The listing builds one solid part. Answer for the finished solid, in the listing's coordinates (mm). A direction names the side the tool comes from. Coordinates: 2 decimals unless noted, no trailing zeros. Order: outer loops, then holes, each group sorted by start corner. A loop starts at its lowest first (then second) coordinate and runs counter-clockwise, first axis right, second up. Notation, with made-up numbers: (29.25, 83.5) -> (83.25, 83.5) arc R12 ccw to (83.25, 103.5) -> close; hole circle Ø1 at (-32.5, 24.25). An arc over 180 degrees is marked (long way). Answer in a Markdown table with one row per item. Add a question column.
```python
from build123d import *

# Parameters (mm, degrees)
SKETCH1_R           = 65
SKETCH1_R_2         = 40
BOSS_EXTRUDE1_DEPTH = 13
SKETCH2_R           = 4.1
CUT_EXTRUDE1_DEPTH  = 93.838569571
SKETCH8_R           = 12
SKETCH8_R_2         = 4.1
BOSS_EXTRUDE4_DEPTH = 13
SKETCH3_W           = 15.2
SKETCH3_H           = 40
SKETCH3_W_2         = 40
SKETCH3_H_2         = 15.2
CUT_EXTRUDE2_DEPTH  = 10.2
BOSS_EXTRUDE2_DEPTH = 13
FILLET1_R           = 30
BOSS_EXTRUDE3_START = -13
BOSS_EXTRUDE3_DEPTH = 13
CUT_EXTRUDE3_DEPTH  = 93.838569571
FILLET2_R           = 30
SKETCH7_OUTSIDE_W   = 168.862
SKETCH7_OUTSIDE_H   = 168.862
CUT_EXTRUDE4_DEPTH  = 93.838569571
FILLET3_R           = 40


with BuildPart() as part:
    # Sketch1 → Boss-Extrude1 (new body)
    with BuildSketch(Plane(origin=(0, 0, 0), x_dir=(1, 0, 0), z_dir=(0, 1, 0))):
        with Locations(Location((0, 0, 0), (0, 0, 90))):
            Circle(SKETCH1_R)
        with Locations(Location((0, 0, 0), (0, 0, 90))):
            Circle(SKETCH1_R_2, mode=Mode.SUBTRACT)
    extrude(amount=BOSS_EXTRUDE1_DEPTH)

    # Sketch2 → Cut-Extrude1 (cut, through all)
    with BuildSketch(Plane(origin=(0, 13, 0), x_dir=(1, 0, 0), z_dir=(0, 1, 0))):
        with Locations(Location((0, 47, 0), (0, 0, 270))):
            Circle(SKETCH2_R)
        with Locations(Location((47, 0, 0), (0, 0, 270))):
            Circle(SKETCH2_R)
        with Locations(Location((0, -47, 0), (0, 0, 270))):
            Circle(SKETCH2_R)
        with Locations(Location((-47, 0, 0), (0, 0, 270))):
            Circle(SKETCH2_R)
    extrude(amount=-CUT_EXTRUDE1_DEPTH, mode=Mode.SUBTRACT)

    # Sketch8 → Boss-Extrude4 (add)
    # profile 1 of 4: a face of its own
    with BuildSketch(Plane(origin=(0, 13, 0), x_dir=(1, 0, 0), z_dir=(0, 1, 0))):
        with Locations((47, 0)):
            Circle(SKETCH8_R)
        with Locations(Location((47, 0, 0), (0, 0, 270))):
            Circle(SKETCH8_R_2, mode=Mode.SUBTRACT)
    # profile 2 of 4: a face of its own
    with BuildSketch(Plane(origin=(0, 13, 0), x_dir=(1, 0, 0), z_dir=(0, 1, 0))):
        with Locations((0, -47)):
            Circle(SKETCH8_R)
        with Locations(Location((0, -47, 0), (0, 0, 270))):
            Circle(SKETCH8_R_2, mode=Mode.SUBTRACT)
    # profile 3 of 4: a face of its own
    with BuildSketch(Plane(origin=(0, 13, 0), x_dir=(1, 0, 0), z_dir=(0, 1, 0))):
        with Locations((-47, 0)):
            Circle(SKETCH8_R)
        with Locations(Location((-47, 0, 0), (0, 0, 270))):
            Circle(SKETCH8_R_2, mode=Mode.SUBTRACT)
    # profile 4 of 4: a face of its own
    with BuildSketch(Plane(origin=(0, 13, 0), x_dir=(1, 0, 0), z_dir=(0, 1, 0))):
        with Locations((0, 47)):
            Circle(SKETCH8_R)
        with Locations(Location((0, 47, 0), (0, 0, 270))):
            Circle(SKETCH8_R_2, mode=Mode.SUBTRACT)
    extrude(amount=-BOSS_EXTRUDE4_DEPTH)

    # Sketch3 → Cut-Extrude2 (cut)
    with BuildSketch(Plane.XZ):
        with Locations((0, 59.6)):
            Rectangle(SKETCH3_W, SKETCH3_H)
        with Locations((59.6, 0)):
            Rectangle(SKETCH3_W_2, SKETCH3_H_2)
        with Locations((0, -59.6)):
            Rectangle(SKETCH3_W, SKETCH3_H)
        with Locations((-59.6, 0)):
            Rectangle(SKETCH3_W_2, SKETCH3_H_2)
    extrude(amount=-CUT_EXTRUDE2_DEPTH, mode=Mode.SUBTRACT)

    # Sketch4 → Boss-Extrude2 (add)
    with BuildSketch(Plane(origin=(0, 13, 0), x_dir=(1, 0, 0), z_dir=(0, 1, 0))):
        Polygon((-33.587572106, -58.336309448), (-58.336309448, -33.587572106), (-56.639196695, -31.890459353), (-31.890459353, -56.639196695), align=None)
    extrude(amount=-BOSS_EXTRUDE2_DEPTH)

    # Fillet1
    # the kernel refuses this fillet: 30 mm, written as the material it adds along each edge
    with BuildSketch(Plane(origin=(-56.639196695, 13, 31.890459353), x_dir=(-0.43072276652908487, 0, -0.9024842926021104), z_dir=(0, -1, 0))) as fillet1_piece_1:
        with BuildLine():
            CenterArc((10.793469922, -29.931661034), FILLET1_R, 93.868064257, 18.866970785)
            Line((-0.800632502, -2.262602703), (-1.032514551, -1.709221536))
            ThreePointArc((-1.032514551, -1.709221536), (-0.965948102, -0.931149887), (-0.565631851, 0.200151465))
            Line((-0.565631851, 0.200151465), (0.040475512, 0.598633221))
            ThreePointArc((0.040475512, 0.598633221), (4.384847156, 0.451932241), (8.729218799, 0.598633221))
            Line((8.729218799, 0.598633221), (8.769694312, 0))
        make_face()
    extrude(amount=13)
    with BuildSketch(Plane(origin=(-31.890459353, 13, 56.639196695), x_dir=(0.9024842926021067, 0, 0.4307227665290924), z_dir=(0, -1, 0))) as fillet1_piece_2:
        with BuildLine():
            CenterArc((10.793469922, 29.931661034), FILLET1_R, 247.264964958, 18.866970785)
            Line((-0.800632502, 2.262602703), (-1.032514551, 1.709221536))
            ThreePointArc((-1.032514551, 1.709221536), (-0.965948102, 0.931149887), (-0.565631851, -0.200151465))
            Line((-0.565631851, -0.200151465), (0.040475512, -0.598633221))
            ThreePointArc((0.040475512, -0.598633221), (4.384847156, -0.451932241), (8.729218799, -0.598633221))
            Line((8.729218799, -0.598633221), (8.769694312, 0))
        make_face()
    extrude(amount=13)

    # Sketch5 → Boss-Extrude3 (add)
    with BuildSketch(Plane(origin=(0, 13, 0), x_dir=(1, 0, 0), z_dir=(0, 1, 0)).offset(BOSS_EXTRUDE3_START)):
        with BuildLine():
            Line((-31.522820305, 59.213121857), (-29.981916204, 57.672217755))
            ThreePointArc((-29.981916204, 57.672217755), (-34.692861997, 54.825243953), (-39.146042554, 51.589899608))
            Line((-39.146042554, 51.589899608), (-31.522820305, 59.213121857))
        make_face()
        with BuildLine():
            Line((-59.213121857, 31.522820305), (-57.672217755, 29.981916204))
            ThreePointArc((-57.672217755, 29.981916204), (-55.348212032, 34.081892918), (-52.733240933, 38.002701228))
            Line((-52.733240933, 38.002701228), (-59.213121857, 31.522820305))
        make_face()
    extrude(amount=BOSS_EXTRUDE3_DEPTH)

    # Sketch6 → Cut-Extrude3 (cut, through all)
    with BuildSketch(Plane(origin=(0, 13, 0), x_dir=(1, 0, 0), z_dir=(0, 1, 0))):
        Polygon((-31.522820305, 59.213121857), (-59.213121857, 31.522820305), (-61.494356901, 33.80405535), (-33.80405535, 61.494356901), align=None)
    extrude(amount=-CUT_EXTRUDE3_DEPTH, mode=Mode.SUBTRACT)

    # Fillet2
    # the kernel refuses this fillet: 30 mm, written as the material it adds along each edge
    with BuildSketch(Plane(origin=(-57.672217755, 0, -29.981916204), x_dir=(-0.4036365927453583, 0, 0.9149193959015831), z_dir=(0, 1, 0))) as fillet2_piece_1:
        with BuildLine():
            CenterArc((10.221339545, -29.938721136), FILLET2_R, 93.662741819, 17.866287174)
            Line((-0.787837769, -2.031768331), (-1.008021315, -1.473629275))
            ThreePointArc((-1.008021315, -1.473629275), (-0.953334813, -0.798965243), (-0.559415929, 0.216918922))
            Line((-0.559415929, 0.216918922), (0.038330023, 0.598774423))
            ThreePointArc((0.038330023, 0.598774423), (4.15241919, 0.467229129), (8.266508357, 0.598774423))
            Line((8.266508357, 0.598774423), (8.304838381, 0))
        make_face()
    extrude(amount=13)
    with BuildSketch(Plane(origin=(-29.981916204, 0, -57.672217755), x_dir=(-0.7071067811865491, 0, -0.7071067811865459), z_dir=(0, 1, 0))) as fillet2_piece_2:
        with BuildLine():
            CenterArc((24.218325876, -20.353758796), FILLET2_R, 137.276688213, 17.866287174)
            Line((-3.002460986, -7.743098124), (-3.546876723, -7.49088491))
            ThreePointArc((-3.546876723, -7.49088491), (-1.936856188, -3.702630997), (-0.572130762, 0.180738462))
            Line((-0.572130762, 0.180738462), (0, 0.6))
            ThreePointArc((0, 0.6), (1.089583739, 0.6), (1.738384311, 0.407075176))
            Line((1.738384311, 0.407075176), (2.179167479, 0))
        make_face()
    extrude(amount=13)

    # Sketch7 outside → Cut-Extrude4 (cut, through all)
    with BuildSketch(Plane(origin=(0, 13, 0), x_dir=(1, 0, 0), z_dir=(0, 1, 0))):
        Rectangle(SKETCH7_OUTSIDE_W, SKETCH7_OUTSIDE_H)
        Polygon((63.245553203, -15), (15, -63.245553203), (-15, -63.245553203), (-63.245553203, -15), (-63.245553203, 15), (-15, 63.245553203), (15, 63.245553203), (63.245553203, 15), align=None, mode=Mode.SUBTRACT)
    extrude(amount=-CUT_EXTRUDE4_DEPTH, mode=Mode.SUBTRACT)

    # Fillet3
    # the kernel refuses this fillet: 40 mm, written as the material it takes off along each edge
    with BuildSketch(Plane(origin=(15, 54.421356237, 63.245553203), x_dir=(-1, 0, 0), z_dir=(0, -1, 0)), Plane(origin=(-15, 54.421356237, 63.245553203), x_dir=(-0.7071067811865475, 0, -0.7071067811865477), z_dir=(0, -1, 0)), Plane(origin=(-63.245553203, 54.421356237, 15), x_dir=(0, 0, -1), z_dir=(0, -1, 0)), Plane(origin=(-63.245553203, 54.421356237, -15), x_dir=(0.7071067811865477, 0, -0.7071067811865475), z_dir=(0, -1, 0)), Plane(origin=(63.245553203, 54.421356237, 15), x_dir=(-0.7071067811865477, 0, 0.7071067811865475), z_dir=(0, -1, 0)), Plane(origin=(63.245553203, 54.421356237, -15), x_dir=(0, 0, 1), z_dir=(0, -1, 0))) as fillet3_piece_1:
        with BuildLine():
            CenterArc((FILLET3_R * 0.414213562373, FILLET3_R), FILLET3_R, 225, 45)
            Line((-FILLET3_R * 0.292893218813, FILLET3_R * 0.292893218813), (0, 0))
            Line((0, 0), (FILLET3_R * 0.414213562373, 0))
        make_face()
    extrude(amount=95.842712475, mode=Mode.SUBTRACT)
    with BuildSketch(Plane(origin=(-15, 54.421356237, -63.245553203), x_dir=(-0.7071067811865476, 0, 0.7071067811865476), z_dir=(0, -1, 0)), Plane(origin=(15, 54.421356237, -63.245553203), x_dir=(-1, 0, 0), z_dir=(0, -1, 0))) as fillet3_piece_2:
        with BuildLine():
            CenterArc((FILLET3_R * 0.414213562373, -FILLET3_R), FILLET3_R, 90, 45)
            Line((-FILLET3_R * 0.292893218813, -FILLET3_R * 0.292893218813), (0, 0))
            Line((0, 0), (FILLET3_R * 0.414213562373, 0))
        make_face()
    extrude(amount=95.842712475, mode=Mode.SUBTRACT)


solid = part.part
```
Q1. Given pin 1 (4 mm diameter, centred on x = 9, y = 8, fed in from -Z); pin 2 (6 mm diameter, centred on y = 2.5, z = 6.5, fed in from +X); pin 3 (5 mm diameter, centred on y = 7, z = -50, fed in from -X), each flat-ended and moving along its own axis, determine where each tip first touches the part or whether it passes through.
Q2. A cutting plane is placed at C-C (z = -22.5). Determine the outline of the cut face in (x, y), then the cut area to 3 significant figures.
Q3. A cutting plane is placed at A-A (x = 21). Determine the outline of the cut face in (y, z).
Q4. A cutting plane is placed at D-D (z = -47). Determine the outline of the cut face in (x, y).
Q5. Straight lines are drawn through the part: line 1 (Z direction, x = -37, y = 12); line 2 (X direction, y = 7.75, z = 0); line 3 (X direction, y = 5.5, z = 30.5). For each, find the intervals that lie inside material, in ascending order.
Q6. For faces 1 (the face through (-52, 10.2, 0)), 2 (the face through (0, 10.2, 52)), 3 (the face through (0, 10.2, -54)), 4 (the face through (28.062, 6.409, 28.505)), determine the directions among +Z, -Z, +X, -X, +Y, -Y from which every point of the face is accessible in a straight line to the end or side of a thin tool.
Q7. Determine the mould class of faces 5 (the face through (39.6, 5, 0)), 6 (the face through (0, 5, 39.6)), 7 (the face through (-36, 13, 0)) for opening direction X: +X half, -X half, draft (parallel to the pull), parting line (faces both ways), or undercut.
Returned:
| question | item | result |
|---|---|---|
| 1 | pin 1 | stops at z = -62.18 |
| 1 | pin 2 | stops at x = 62.18 |
| 1 | pin 3 | stops at x = -30.75 |
| 2 | outline | (-55.19, 0) -> (-33.07, 0) -> (-33.07, 13) -> (-55.19, 13) -> close; (33.07, 0) -> (55.19, 0) -> (55.19, 13) -> (33.07, 13) -> close |
| 2 | area | 575 mm² |
| 3 | outline | (0, -56.27) -> (13, -56.27) -> (13, -34.04) -> (0, -34.04) -> close; (0, 34.04) -> (13, 34.04) -> (13, 56.27) -> (0, 56.27) -> close |
| 4 | outline | (-31.25, 0) -> (-7.6, 0) -> (-7.6, 10.2) -> (-4.1, 10.2) -> (-4.1, 13) -> (-31.25, 13) -> close; (4.1, 10.2) -> (7.6, 10.2) -> (7.6, 0) -> (31.25, 0) -> (31.25, 13) -> (4.1, 13) -> close |
| 5 | line 1 | z = -41.25 to -15.2, -6.63 to 6.63, 15.2 to 41.25 |
| 5 | line 2 | x = -39.6 to -35, 35 to 39.6 |
| 5 | line 3 | x = -47.75 to -25.88, 25.88 to 47.75 |
| 6 | face 1 | -X, -Y |
| 6 | face 2 | +Z, -Y |
| 6 | face 3 | -Z, -Y |
| 6 | face 4 | +Y, -Y |
| 7 | face 5 | +X half |
| 7 | face 6 | undercut |
| 7 | face 7 | draft |
